```python
from build123d import *

# Parameters (mm, degrees)
ESQUISSE1_R                  = 36
BASE_EXTRUSION_DEPTH         = 8
ESQUISSE2_R                  = 32.5
BOSS_EXTRU_1_DEPTH           = 4
ESQUISSE4_R                  = 28
BOSS_EXTRU_2_DEPTH           = 9
ESQUISSE5_R                  = 31.8
BOSS_EXTRU_3_DEPTH           = 7.5
ESQUISSE6_R                  = 18
ENL_V_MAT_EXTRU_1_DEPTH      = 52.5
ESQUISSE10_W                 = 20
ESQUISSE10_H                 = 14.61003861
ENL_V_MAT_EXTRU_5_DEPTH      = 52.5
R_P_TITION_CIRCULAIRE1_COUNT = 4
ESQUISSE13_R                 = 4.5
ENL_V_MAT_EXTRU_6_DEPTH      = 37
ENL_V_MAT_EXTRU_6_DEPTH_BACK = 37
ENL_V_START                  = -31.8
ESQUISSE14_R                 = 1.23
ENL_V_MAT_EXTRU_7_DEPTH      = 13.842074
R_P_TITION_CIRCULAIRE2_COUNT = 2
R_P_TITION_CIRCULAIRE2_ANGLE = 120


with BuildPart() as part:
    # Esquisse1 → Base-Extrusion (new body)
    with BuildSketch(Plane.XY):
        Circle(ESQUISSE1_R)
    extrude(amount=BASE_EXTRUSION_DEPTH)

    # Esquisse2 → Boss.-Extru.1 (add)
    with BuildSketch(Plane(origin=(0, 0, 0), x_dir=(-1, 0, 0), z_dir=(0, 0, -1))):
        Circle(ESQUISSE2_R)
    extrude(amount=BOSS_EXTRU_1_DEPTH)

    # Esquisse3 → Boss.-Révol.1 (revolve)
    with BuildSketch(Plane(origin=(0, 0, 0), x_dir=(0, 0, -1), z_dir=(1, 0, 0))):
        Polygon((4, 32.5), (27, 22.499315376), (27, 0), (4, 0), align=None)
    revolve(axis=Axis((0, 0, 0), (0, 0, -1)))

    # Esquisse4 → Boss.-Extru.2 (add)
    with BuildSketch(Plane.XY.offset(8)):
        with Locations((0, 3)):
            Circle(ESQUISSE4_R)
    extrude(amount=BOSS_EXTRU_2_DEPTH)

    # Esquisse5 → Boss.-Extru.3 (add)
    with BuildSketch(Plane.XY.offset(17)):
        with Locations((0, 3)):
            Circle(ESQUISSE5_R)
    extrude(amount=BOSS_EXTRU_3_DEPTH)

    # Esquisse6 → Enlèv. mat.-Extru.1 (cut, through all)
    with BuildSketch(Plane.XY.offset(24.5)):
        with Locations((0, 3)):
            Circle(ESQUISSE6_R)
    extrude(amount=-ENL_V_MAT_EXTRU_1_DEPTH, mode=Mode.SUBTRACT)

    # Esquisse10 → Enlèv. mat.-Extru.5 (cut, through all)
    with BuildSketch(Plane.XY.offset(24.5)):
        with Locations((0, 31.305019305)):
            Rectangle(ESQUISSE10_W, ESQUISSE10_H)
    extrude(amount=-ENL_V_MAT_EXTRU_5_DEPTH, mode=Mode.SUBTRACT)

    # Esquisse11 → Perçage1 (revolve, cut)
    with BuildSketch(Plane(origin=(-17.67766953, 20.67766953, 24.5), x_dir=(0, -1, 0), z_dir=(1, 0, 0))):
        Polygon((0, 0), (0, 12.976398506), (1.625, 12), (1.625, 0), align=None)
    per_age1 = revolve(axis=Axis((-17.67766953, 20.67766953, 28.744199587), (0, 0, -1)), mode=Mode.SUBTRACT)

    # Répétition circulaire1: Perçage1 ×4 about axis
    r_p_tition_circulaire1_axis = Axis((0, 3, 0), (0, 0, 1))
    for i in range(1, R_P_TITION_CIRCULAIRE1_COUNT):
        add(per_age1.rotate(r_p_tition_circulaire1_axis, i * 360 / R_P_TITION_CIRCULAIRE1_COUNT), mode=Mode.SUBTRACT)

    # Esquisse13 → Enlèv. mat.-Extru.6 (cut, two sides)
    with BuildSketch(Plane(origin=(0, 0, 0), x_dir=(0, 0, -1), z_dir=(1, 0, 0))) as enl_v_mat_extru_6_sk:
        with Locations((-12.5, 3)):
            Circle(ESQUISSE13_R)
    extrude(amount=ENL_V_MAT_EXTRU_6_DEPTH, mode=Mode.SUBTRACT)
    extrude(enl_v_mat_extru_6_sk.sketch, amount=-ENL_V_MAT_EXTRU_6_DEPTH_BACK, mode=Mode.SUBTRACT)

    # Esquisse14 → Enlèv. mat.-Extru.7 (cut)
    with BuildSketch(Plane(origin=(-1.299038106, 0.75, 0), x_dir=(0, 0, 1), z_dir=(-0.866025404, 0.5, 0)).offset(ENL_V_START)):
        with Locations((20.75, 2.598076211)):
            Circle(ESQUISSE14_R)
    enl_v_mat_extru_7 = extrude(amount=ENL_V_MAT_EXTRU_7_DEPTH, mode=Mode.SUBTRACT)

    # Répétition circulaire2: Enlèv. mat.-Extru.7 ×2 about axis
    r_p_tition_circulaire2_axis = Axis((0, 3, 0), (0, 0, -1))
    for i in range(1, R_P_TITION_CIRCULAIRE2_COUNT):
        add(enl_v_mat_extru_7.rotate(r_p_tition_circulaire2_axis, i * R_P_TITION_CIRCULAIRE2_ANGLE / (R_P_TITION_CIRCULAIRE2_COUNT - 1)), mode=Mode.SUBTRACT)

    # Esquisse16 → Révolution1 (revolve)
    with BuildSketch(Plane(origin=(0, 0, 0), x_dir=(0, 0, -1), z_dir=(1, 0, 0))):
        Polygon((27, -15), (27, -13), (17, -13), (17, -11), (4, -11), (4, -13), (-4, -13), (-4, -15), align=None)
    revolve(axis=Axis((0, 3, -27), (0, 0, 1)))


solid = part.part
```
CAD build for the part. Positions are in the model's coordinates, mm. A direction names the side the tool comes from. Round coordinates to 2 decimals unless told otherwise and drop trailing zeros. Order: outer loops, then holes, each group sorted by start corner. A loop starts at its lowest first (then second) coordinate and runs counter-clockwise, first axis right, second up. Notation, with made-up numbers: (16.25, 73) - (30.25, 73) arc R6 cw to (30.25, 84) - close; hole circle Ø11 at (6, 82.5). An arc over 180 degrees is marked (long way). Answer in a Markdown table with one row per item. Add a question column.
(1) Band-saw the part on B-B on z = 15. List the corners of the cut face in (x, y) (3 decimals).
(2) Probe L1, parallel to X at y = 3, z = 20; L2, parallel to Y at x = 0, z = 9; L3, parallel to Y at x = 2.5, z = -23.5. List the from-to ranges inside material, lowest first. Write a range as [from, to].
(3) Band-saw the part on D-D on y = 0. Count the separate pieces of the cut face and the enclosed holes in it, and give its area (3 significant figures).
(4) 3-axis set-ups, long thin cutter, end or side, ignore diameter. For faces 4 (the face through (16.236, -13.928, 18.584)), 5 (the face through (23.2, 18.68, 12.44)), 6 (the face through (2, -27, 8)): which of +Z, -Z, +X, -X, +Y, -Y reach the whole face in a straight line?
(5) Drop flat-ended pins along their axis: pin 1 Ø2 at (x, z) = (13.5, -10.5) entering from -Y; pin 2 Ø8 at (x, z) = (21, 1) entering from -Y; pin 3 Ø16 at (x, y) = (5.5, 8) entering from +Z. Give the stop position or say it passes through.
(6) Band-saw the part on C-C on z = -8.5. List the corners of the cut face in (x, y), and give its area (3 significant figures).
(7) Band-saw the part on A-A on x = 0. List the corners of the cut face in (y, z), and give its area (3 significant figures).
(8) Mould opens along Y. For faces 1 (the face through (1.287, -32.475, -1.972)), 2 (the face through (-17.96, -14.69, 11.693)), 3 (the face through (-22.93, 19.07, 12.44)) say: +Y half, -Y half, draft (parallel to the pull), parting line (faces both ways), or undercut.
Data:
| question | item | result |
|---|---|---|
| 1 | outline | (-27.749, -0.742) arc R28 ccw to (27.749, -0.742) - (17.607, -0.742) arc R18 cw to (-17.607, -0.742) - close; (-27.749, 6.742) - (-17.607, 6.742) arc R18 cw to (17.607, 6.742) - (27.749, 6.742) arc R28 ccw to (10, 29.153) - (10, 24) - (-10, 24) - (-10, 29.153) arc R28 ccw to start; hole circle Ø3.25 at (-17.678, -14.678); hole circle Ø3.25 at (-17.678, 20.678); hole circle Ø3.25 at (17.678, -14.678); hole circle Ø3.25 at (17.678, 20.678) |
| 2 | L1 | x = [-31.8, -18], [18, 31.8] |
| 2 | L2 | y = [-25, -15], [21, 24] |
| 2 | L3 | y = [-23.89, -12.8], [18.8, 23.89] |
| 3 | separate pieces | 4 |
| 3 | enclosed holes | 0 |
| 3 | area | 1,290 mm^2 |
| 4 | face 4 | +Z |
| 4 | face 5 | +X, +Y |
| 4 | face 6 | none |
| 5 | pin 1 | stops at y = -27.11 |
| 5 | pin 2 | stops at y = -31.73 |
| 5 | pin 3 | stops at z = -4 |
| 6 | outline | (-10, 24) - (-10, 28.86) arc R30.54 ccw (long way) to (10, 28.86) - (10, 24) - close; hole circle Ø28 at (0, 3) |
| 6 | area | 2,200 mm^2 |
| 7 | outline | (-36, 0) - (-32.5, 0) - (-32.5, -4) - (-22.5, -27) - (-13, -27) - (-13, -17) - (-11, -17) - (-11, -4) - (-13, -4) - (-13, 4) - (-15, 4) - (-15, 24.5) - (-28.8, 24.5) - (-28.8, 17) - (-25, 17) - (-25, 8) - (-36, 8) - close; (17, -17) - (19, -17) - (19, -27) - (22.5, -27) - (24, -23.55) - (24, 24.5) - (21, 24.5) - (21, 4) - (19, 4) - (19, -4) - (17, -4) - close |
| 7 | area | 1,050 mm^2 |
| 8 | face 1 | parting line |
| 8 | face 2 | undercut |
| 8 | face 3 | +Y half |
